Input: part model. Units: mm. Frame: model coordinates. A direction names the side the tool comes from. Give positions to 0.01 mm unless a question says otherwise; leave off trailing zeros. Loops run counter-clockwise (first coordinate to the right, second up) from the corner with the lowest first, then second, coordinate; pieces in that order, holes last. Notation, with made-up numbers: (58.25, 3) -> (106.25, 3) arc R12 cw to (106.25, 20) -> close; hole circle Ø1 at (-3.75, -5). An arc over 180 degrees is marked (long way). Answer as a JSON object with one key per item and string values.
```python
from build123d import *

# Parameters (mm, degrees)
BOSS_EXTRU_1_DEPTH = 3
CONG_1_R           = 0.1
BOSS_EXTRU_2_DEPTH = 1.5
CONG_2_R           = 0.2
CONG_3_R           = 0.1


with BuildPart() as part:
    # Esquisse1 → Boss.-Extru.1 (new body)
    with BuildSketch(Plane.XY):
        with BuildLine():
            ThreePointArc((-8.03233352, 17.581173717), (-1.821522293, -1.442775514), (9.198940383, -18.147093005))
            Line((9.198940383, -18.147093005), (-4.524586287, -18.147093005))
            ThreePointArc((-4.524586287, -18.147093005), (-5.134783325, -17.939342697), (-5.491443118, -17.402412154))
            ThreePointArc((-5.491443118, -17.402412154), (-8.390456717, -0.028903657), (-8.03233352, 17.581173717))
        make_face()
        with BuildLine():
            ThreePointArc((-7.54889357, 10.99150579), (-7.101772019, -3.192262147), (-4.524586287, -17.147093005))
            Line((-4.524586287, -17.147093005), (7.041670832, -17.147093005))
            ThreePointArc((7.041670832, -17.147093005), (-1.736845674, -3.846887542), (-7.54889357, 10.99150579))
        make_face(mode=Mode.SUBTRACT)
    extrude(amount=BOSS_EXTRU_1_DEPTH)

    # Cong_1
    cong_1_edges = [part.edges().sort_by_distance(p)[0] for p in [
        (-8.03233352, 17.581173717, 1.5),
    ]]
    fillet(cong_1_edges, radius=CONG_1_R)

    # Esquisse2 → Boss.-Extru.2 (add)
    with BuildSketch(Plane.XY.offset(3)):
        with BuildLine():
            Line((-4.524586287, -20.147093005), (13.781531415, -20.147093005))
            ThreePointArc((13.781531415, -20.147093005), (1.144889736, -2.883958877), (-5.944425785, 17.301236646))
            ThreePointArc((-5.944425785, 17.301236646), (-8.095151796, 19.001327524), (-10.094549972, 17.125604115))
            ThreePointArc((-10.094549972, 17.125604115), (-10.359767763, -0.515611426), (-7.425156781, -17.913050452))
            ThreePointArc((-7.425156781, -17.913050452), (-6.355177402, -19.523842081), (-4.524586287, -20.147093005))
        make_face()
        with BuildLine():
            Line((-4.524586287, -17.147093005), (7.041670832, -17.147093005))
            ThreePointArc((7.041670832, -17.147093005), (-1.736845674, -3.846887542), (-7.54889357, 10.99150579))
            ThreePointArc((-7.54889357, 10.99150579), (-7.101772019, -3.192262147), (-4.524586287, -17.147093005))
        make_face(mode=Mode.SUBTRACT)
    extrude(amount=BOSS_EXTRU_2_DEPTH)

    # Cong_2
    cong_2_edges = [part.edges().sort_by_distance(p)[0] for p in [
        (13.781531415, -20.147093005, 3.75),
    ]]
    fillet(cong_2_edges, radius=CONG_2_R)

    # Cong_3
    cong_3_edges = [part.edges().sort_by_distance(p)[0] for p in [
        (9.198940383, -18.147093005, 1.5),
    ]]
    fillet(cong_3_edges, radius=CONG_3_R)


solid = part.part
```
Q1. Section B-B, the plane z = 3.8. Return the cut outline in (x, y).
Evaluation:
{"outline": "(-10.09, 17.13) arc R97 ccw to (-7.43, -17.91) arc R3 ccw to (-4.52, -20.15) -> (13.31, -20.15) arc R0.2 ccw to (13.45, -19.81) arc R73 cw to (-5.94, 17.3) arc R2.1 ccw to start; hole (-7.55, 10.99) arc R94 ccw to (-4.52, -17.15) -> (7.04, -17.15) arc R76 cw to start"}
Q2. Section D-D, the plane y = 13. Return the cut outline in (x, z).
Evaluation:
{"outline": "(-10.45, 3) -> (-8.44, 3) -> (-8.44, 0) -> (-7.04, 0) -> (-7.04, 3) -> (-4.98, 3) -> (-4.98, 4.5) -> (-10.45, 4.5) -> close"}
Q3. Access query for faces 1 (the flat face through (2, -18.147, 1)), 2 (the cylindrical face through (-5.127, -17.945, 1.479)), 3 (the cylindrical face through (-8.347, -0.605, 1.479)). Directions: +Z, -Z, +X, -X, +Y, -Y. A direction counts if a zero-diameter tool reaches every point of the face in a straight line with its end or side. Return the directions, or none.
Evaluation:
{"face 1": "-Z, +X, -X, -Y", "face 2": "-Z, -X, -Y", "face 3": "-Z, -X"}
Q4. Section A-A, the plane y = 7.5. Return the cut outline in (x, z), then the cut area to 3 significant figures.
Evaluation:
{"outline": "(-10.64, 3) -> (-8.64, 3) -> (-8.64, 0) -> (-7.64, 0) -> (-7.64, 4.5) -> (-10.64, 4.5) -> close; (-6.5, 0) -> (-5.45, 0) -> (-5.45, 3) -> (-3.33, 3) -> (-3.33, 4.5) -> (-6.5, 4.5) -> close", "area": "15.4 mm2"}
Q5. Pin query (flat end, axial travel): pin 1 (2 mm diameter, centred on x = 8, z = 1.5, fed in from -Y). Return the tip coordinate at first contact, or that it passes through.
Evaluation:
{"pin 1": "stops at y = -18.15"}
Q6. Draft query along X for faces 4 (the cylindrical face through (-10.38, -0.27, 3.74)), 5 (the cylindrical face through (-1.84, -1.4, 1.48)), 6 (the flat face through (-1, -3, 4.5)), 7 (the cylindrical face through (-1.63, -4.05, 2.22)). Return one class per face: +X half, -X half, draft (parallel to the pull), parting line (faces both ways), or undercut.
Evaluation:
{"face 4": "-X half", "face 5": "+X half", "face 6": "draft", "face 7": "undercut"}
Q7. Ray query, line 1 along Y through (x, z) = (0.75, 3.45); line 2 along Y through (x, z) = (6, 2.75); line 3 along X through (y, z) = (6, 3.7). Return the intervals inside material, ascending.
Evaluation:
{"line 1": "y = -20.15 to -17.15, -8.27 to -2.12", "line 2": "y = -18.15 to -17.15, -15.85 to -14.22", "line 3": "x = -10.64 to -7.64, -5.99 to -2.8"}
Q8. Section C-C, the plane x = 5.75. Return the cut outline in (y, z), then the cut area to 3 significant figures.
Evaluation:
{"outline": "(-20.15, 3) -> (-18.15, 3) -> (-18.15, 0) -> (-17.15, 0) -> (-17.15, 4.5) -> (-20.15, 4.5) -> close; (-15.53, 0) -> (-13.89, 0) -> (-13.89, 3) -> (-10.47, 3) -> (-10.47, 4.5) -> (-15.53, 4.5) -> close", "area": "20.0 mm2"}
